from build123d import *

# Parameters (mm, degrees)
CROQUIS1_R              = 4
SALIENTE_EXTRUIR1_DEPTH = 6


with BuildPart() as part:
    # Croquis1 → Saliente-Extruir1 (new body)
    with BuildSketch(Plane.XY):
        Polygon((-560, 30), (-600, 30), (-648, 30), (-648, -19), (-630, -110), (-600, -110), (-550, -110), (-470, -30), (470, -30), (550, -110), (600, -110), (630, -110), (648, -19), (648, 30), (600, 30), (560, 30), align=None)
        with Locations((-615.3, 0)):
            Circle(CROQUIS1_R, mode=Mode.SUBTRACT)
        with BuildLine():
            ThreePointArc((-544.7, -4), (-548.7, 0), (-544.7, 4))
            Line((-544.7, 4), (-534.7, 4))
            ThreePointArc((-534.7, 4), (-530.7, 0), (-534.7, -4))
            Line((-534.7, -4), (-544.7, -4))
        make_face(mode=Mode.SUBTRACT)
        with BuildLine():
            ThreePointArc((544.7, 4), (548.7, 0), (544.7, -4))
            Line((544.7, -4), (534.7, -4))
            ThreePointArc((534.7, -4), (530.7, 0), (534.7, 4))
            Line((534.7, 4), (544.7, 4))
        make_face(mode=Mode.SUBTRACT)
        with Locations((615.3, 0)):
            Circle(CROQUIS1_R, mode=Mode.SUBTRACT)
    extrude(amount=SALIENTE_EXTRUIR1_DEPTH)


solid = part.part
Design review of the part built by this model. Coordinates are the model's own, in mm. A direction names the side the tool comes from. Coordinates: 2 decimals unless noted, no trailing zeros. Loops run counter-clockwise (first coordinate to the right, second up) from the corner with the lowest first, then second, coordinate; pieces in that order, holes last. Notation, with made-up numbers: M 11.25,61.25 L 24.25,61.25 A34 cw 24.25,97.25 Z; hole C 89.5,74 d4. An arc over 180 degrees is marked long. Answer as CSV lines item,"result".
Item 1: The part is to be moulded in two halves that separate along X. For faces 3 (the face through (-9, -8, 0)), 4 (the face through (509, -69, 3)), say which applies: pulls with the +X half, pulls with the -X half, needs draft (parallel to the pull), parting line crosses it, or undercut.
Answer list:
face 3,"needs draft"
face 4,"undercut"
Item 2: For probe 1 along Y at (x, z) = (615.3, 3.7); probe 2 along Y at (x, z) = (160.5, 4.55); probe 3 along X at (y, z) = (-62, 5.3), list the stretches that pass through material, from the lowest coordinate up.
Answer list:
probe 1,"-110 to -4, 4 to 30"
probe 2,"-30 to 30"
probe 3,"-639.49 to -502, 502 to 639.49"
Item 3: Add section C-C on x = -228. State the section outline as (y, z) points, plus the area to 3 significant figures.
Answer list:
outline,"M -30,0 L 30,0 L 30,6 L -30,6 Z"
area,"360 mm²"
Item 4: For P1, Ø3, axis at x = 136, z = 4, coming from the -Y side; P2, Ø5, axis at x = -615.3, y = 0, coming from the -Z side, all flat-tipped, find the tip position at first contact; note any pin that passes through.
Answer list:
P1,"y = -30"
P2,"through"
Item 5: Add section B-B on y = -48.5. State the section outline as (x, z) points, plus the area to 3 significant figures.
Answer list:
outline,"M -642.16,0 L -488.5,0 L -488.5,6 L -642.16,6 Z; M 488.5,0 L 642.16,0 L 642.16,6 L 488.5,6 Z"
area,"1,840 mm²"
Item 6: Machinability: for faces 1 (the face through (-9, -8, 6)), 2 (the face through (-511, -71, 3)), which of the approach directions +Z, -Z, +X, -X, +Y, -Y give a long, thin tool a straight path to every point of the face, cutting with its end or side? Answer none if there is none.
Answer list:
face 1,"+Z, +X, -X, +Y, -Y"
face 2,"+Z, -Z, -Y"
Item 7: Add section A-A on z = 3.4. State the section outline as (x, y) points, plus the area to 3 significant figures.
Answer list:
outline,"M -648,-19 L -630,-110 L -550,-110 L -470,-30 L 470,-30 L 550,-110 L 630,-110 L 648,-19 L 648,30 L -648,30 Z; hole C -615.3,0 d8; hole M -544.7,-4 L -534.7,-4 A4 ccw -534.7,4 L -544.7,4 A4 ccw Z; hole M 534.7,-4 L 544.7,-4 A4 ccw 544.7,4 L 534.7,4 A4 ccw Z; hole C 615.3,0 d8"
area,"97,800 mm²"
